Verification items for this drawing (mm, ordinates from the low corner). Coordinates: 2 decimals unless noted, no trailing zeros. Order: outer loops, then holes, each group sorted by start corner. A loop starts at its lowest first (then second) coordinate and runs counter-clockwise, first axis right, second up.
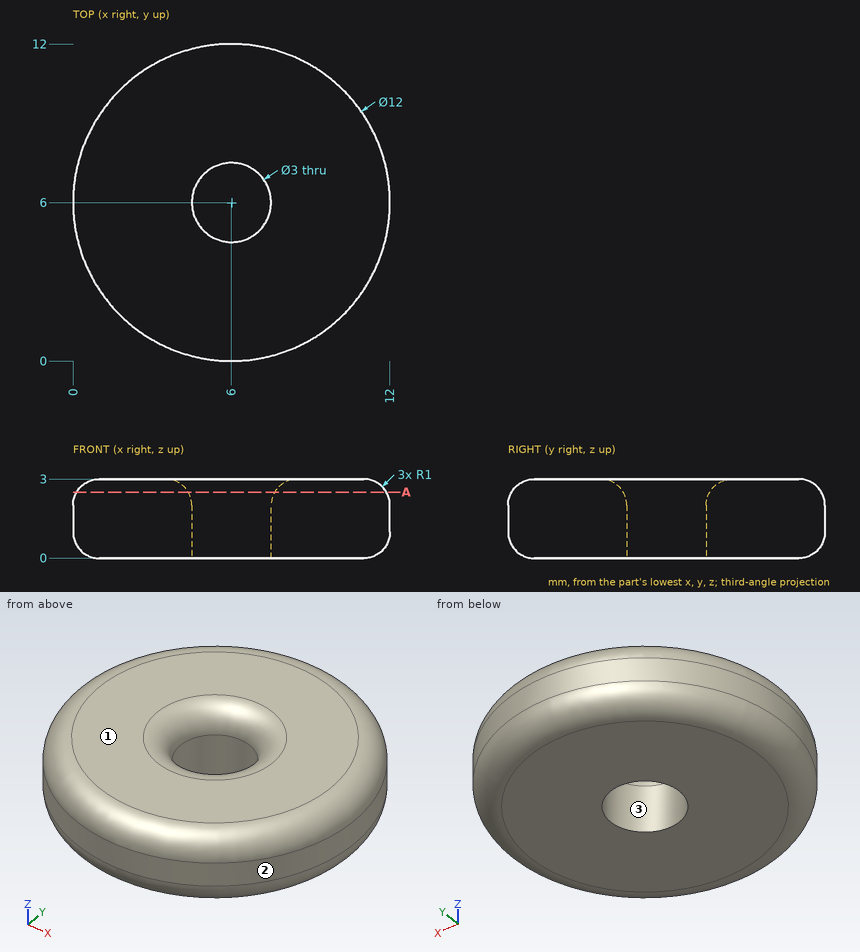
Item 1: Thickness scan on line 1 along Y through (x, z) = (6, 1.05); line 2 along Y through (x, z) = (6, 0.55); line 3 along X through (y, z) = (5.25, 1.8). Record the ranges inside material, lowest first.
Item 2: Release check for a two-part mould opening along Y. For the marked faces 1, 2 and 3 record: pulls with the +Y half, pulls with the -Y half, needs draft (parallel to the pull), parting line crosses it, or undercut.
Item 3: Depth check by flat-ended pin: P1, Ø1.8, axis at x = 6, y = 6, coming from the -Z side; P2, Ø1.5, axis at x = 3, z = 1, coming from the -Y side. Enter the tip coordinate at first touch or a pass-through.
Item 4: Sectioned sample at A-A (z = 2.5). Record the cut outline in (x, y), and give its area (3 significant figures).
Geometry check:
1. line 1: y = 0 to 4.5, 7.5 to 12
1. line 2: y = 0.11 to 4.5, 7.5 to 11.89
1. line 3: x = 0.05 to 4.7, 7.3 to 11.95
2. face 1: needs draft
2. face 2: parting line crosses it
2. face 3: undercut
3. P1: passes through
3. P2: stops at y = 0.44
4. outline: circle Ø11.73 at (6, 6); hole circle Ø3.27 at (6, 6)
4. area: 99.7 mm2
